Part model, mm, in its own coordinate system. A direction names the side the tool comes from. Coordinates: 2 decimals unless noted, no trailing zeros. Write each loop counter-clockwise with the first axis right and the second up, starting at its lowest first coordinate (ties: lowest second). Pieces come first, ordered by that corner, then holes. Notation, with made-up numbers: (25, 73.25) -> (64, 73.25) arc R27 cw to (64, 98.25) -> close; hole circle Ø9 at (27.5, -22.75). An arc over 180 degrees is marked (long way). Write item = value, one per line.
from build123d import *

# Parameters (mm, degrees)
SKETCH1_W           = 91
SKETCH1_H           = 24
BOSS_EXTRUDE1_DEPTH = 4
SKETCH2_R           = 1.675
CUT_EXTRUDE1_DEPTH  = 48.22552276
SKETCH3_W           = 91
SKETCH3_H           = 6
CUT_EXTRUDE2_DEPTH  = 2.5
SKETCH4_W           = 91
SKETCH4_H           = 4
BOSS_EXTRUDE2_DEPTH = 2.2
SKETCH5_W           = 91
SKETCH5_H           = 2
BOSS_EXTRUDE3_DEPTH = 17.62
SKETCH6_R           = 1.75
CUT_EXTRUDE3_DEPTH  = 55.464248824
SKETCH7_W           = 91
SKETCH7_H           = 24.2
SKETCH7_R           = 1.675
BOSS_EXTRUDE5_DEPTH = 2
SKETCH8_W           = 91
SKETCH8_H           = 6
BOSS_EXTRUDE6_DEPTH = 1
CHAMFER1_SIZE       = 0.7
FILLET1_R           = 3


with BuildPart() as part:
    # Sketch1 → Boss-Extrude1 (new body)
    with BuildSketch(Plane(origin=(0, 0, 0), x_dir=(1, 0, 0), z_dir=(0, 1, 0))):
        Rectangle(SKETCH1_W, SKETCH1_H)
    extrude(amount=BOSS_EXTRUDE1_DEPTH)

    # Sketch2 → Cut-Extrude1 (cut, through all)
    with BuildSketch(Plane(origin=(0, 4, 0), x_dir=(1, 0, 0), z_dir=(0, 1, 0))):
        with Locations(Location((-40.6, 3.5, 0), (0, 0, 270))):
            Circle(SKETCH2_R)
        with Locations(Location((-40.6, -9.95, 0), (0, 0, 270))):
            Circle(SKETCH2_R)
        with Locations(Location((40.6, 3.5, 0), (0, 0, 270))):
            Circle(SKETCH2_R)
        with Locations(Location((40.6, -9.95, 0), (0, 0, 270))):
            Circle(SKETCH2_R)
    extrude(amount=-CUT_EXTRUDE1_DEPTH, mode=Mode.SUBTRACT)

    # Sketch3 → Cut-Extrude2 (cut)
    with BuildSketch(Plane(origin=(0, 4, 0), x_dir=(1, 0, 0), z_dir=(0, 1, 0))):
        with Locations((0, -3.65)):
            Rectangle(SKETCH3_W, SKETCH3_H)
    extrude(amount=-CUT_EXTRUDE2_DEPTH, mode=Mode.SUBTRACT)

    # Sketch4 → Boss-Extrude2 (add)
    with BuildSketch(Plane(origin=(0, 0, -12), x_dir=(-1, 0, 0), z_dir=(0, 0, -1))):
        with Locations((0, 2)):
            Rectangle(SKETCH4_W, SKETCH4_H)
    extrude(amount=BOSS_EXTRUDE2_DEPTH)

    # Sketch5 → Boss-Extrude3 (add)
    with BuildSketch(Plane.XZ):
        with Locations((0, -13.2)):
            Rectangle(SKETCH5_W, SKETCH5_H)
    extrude(amount=BOSS_EXTRUDE3_DEPTH)

    # Sketch6 → Cut-Extrude3 (cut, through all)
    with BuildSketch(Plane.XY.offset(-12.2)):
        with Locations((-21.25, -10.12)):
            Circle(SKETCH6_R)
        with Locations((0, -10.12)):
            Circle(SKETCH6_R)
        with Locations((21.25, -10.12)):
            Circle(SKETCH6_R)
    extrude(amount=-CUT_EXTRUDE3_DEPTH, mode=Mode.SUBTRACT)

    # Sketch7 → Boss-Extrude5 (add)
    with BuildSketch(Plane.XZ):
        with Locations((0, -0.1)):
            Rectangle(SKETCH7_W, SKETCH7_H)
        with Locations(Location((40.6, 9.95, 0), (0, 0, 90))):
            Circle(SKETCH7_R, mode=Mode.SUBTRACT)
        with Locations(Location((40.6, -3.5, 0), (0, 0, 90))):
            Circle(SKETCH7_R, mode=Mode.SUBTRACT)
        with Locations(Location((-40.6, -3.5, 0), (0, 0, 90))):
            Circle(SKETCH7_R, mode=Mode.SUBTRACT)
        with Locations(Location((-40.6, 9.95, 0), (0, 0, 90))):
            Circle(SKETCH7_R, mode=Mode.SUBTRACT)
    extrude(amount=BOSS_EXTRUDE5_DEPTH)

    # Sketch8 → Boss-Extrude6 (add)
    with BuildSketch(Plane.XY.offset(12)):
        with Locations((0, 1)):
            Rectangle(SKETCH8_W, SKETCH8_H)
    extrude(amount=BOSS_EXTRUDE6_DEPTH)

    # Chamfer1
    chamfer1_edges = [part.edges().sort_by_distance(p)[0] for p in [
        (40.6, 4, 8.275),
        (-40.6, 4, -5.175),
        (40.6, 4, -5.175),
        (-40.6, 4, 8.275),
    ]]
    chamfer(chamfer1_edges, length=CHAMFER1_SIZE)

    # Fillet1
    fillet1_edges = [part.edges().sort_by_distance(p)[0] for p in [
        (0, -2, -12.2),
    ]]
    fillet(fillet1_edges, radius=FILLET1_R)


solid = part.part
Q1. Saw through at C-C on y = -10.12. Give the cut face in (x, z).
Model answer:
outline = (-45.5, -14.2) -> (-23, -14.2) -> (-23, -12.2) -> (-45.5, -12.2) -> close; (-19.5, -14.2) -> (-1.75, -14.2) -> (-1.75, -12.2) -> (-19.5, -12.2) -> close; (1.75, -14.2) -> (19.5, -14.2) -> (19.5, -12.2) -> (1.75, -12.2) -> close; (23, -14.2) -> (45.5, -14.2) -> (45.5, -12.2) -> (23, -12.2) -> close
Q2. Saw through at B-B on x = -40.6. Give the cut face in (y, z) (3 decimals), and give its area (3 significant figures).
Model answer:
outline = (-17.62, -14.2) -> (4, -14.2) -> (4, -5.875) -> (3.3, -5.175) -> (-2, -5.175) -> (-2, -9.2) arc R3 cw to (-5, -12.2) -> (-17.62, -12.2) -> close; (-2, -1.825) -> (3.3, -1.825) -> (4, -1.125) -> (4, 0.65) -> (1.5, 0.65) -> (1.5, 6.65) -> (4, 6.65) -> (4, 7.575) -> (3.3, 8.275) -> (-2, 8.275) -> close; (-2, 11.625) -> (3.3, 11.625) -> (4, 12.325) -> (4, 13) -> (-2, 13) -> close
area = 140 mm²
Q3. Pin check, flat tips, straight feed: pin 1 (2 mm diameter, centred on x = -34, z = -3, fed in from -Y); pin 2 (12 mm diameter, centred on x = 2.5, z = -10.5, fed in from -Y); pin 3 (3 mm diameter, centred on x = -22, z = 3.5, fed in from +Y); pin 4 (5.5 mm diameter, centred on x = 21.25, y = -10.12, fed in from +Z). Stop position of each tip, or through.
Model answer:
pin_1 = -2
pin_2 = -17.62
pin_3 = 1.5
pin_4 = -12.2
Q4. Saw through at A-A on z = 9.95. Give the cut face in (x, y) (3 decimals).
Model answer:
outline = (-45.5, -2) -> (-42.275, -2) -> (-42.275, 3.3) -> (-42.975, 4) -> (-45.5, 4) -> close; (-38.925, -2) -> (38.925, -2) -> (38.925, 3.3) -> (38.225, 4) -> (-38.225, 4) -> (-38.925, 3.3) -> close; (42.275, -2) -> (45.5, -2) -> (45.5, 4) -> (42.975, 4) -> (42.275, 3.3) -> close
Q5. Which spindle directions (+Z, -Z, +X, -X, +Y, -Y) get a long thin tool onto all of the face, cutting with end or side? Do faces 5 (the face through (-1, -7, -14.2)), 6 (the face through (-1, -2, 2)), 7 (the face through (-1, 3, 0.65)). Say none if no direction does.
Model answer:
face_5 = -Z, +X, -X, +Y, -Y
face_6 = +Z, +X, -X, -Y
face_7 = +X, -X, +Y
Q6. Probe line 1 (X direction, y = 1.7, z = -3.5) (3 decimals); line 2 (Z direction, x = -40.6, y = 1) (3 decimals); line 3 (Y direction, x = 21.25, z = -12.9). List the from-to ranges inside material, lowest first. Write a range as from..to.
Model answer:
line_1 = -45.5..-42.275, -38.925..38.925, 42.275..45.5
line_2 = -14.2..-5.175, -1.825..8.275, 11.625..13
line_3 = -17.62..-11.87, -8.37..4
Q7. Mould opens along Z. For faces 1 (the face through (-1, 4, 10)), 2 (the face through (0.64, -2.86, -11.3)), 3 (the face through (-1, 3, 6.65)), 4 (the face through (-39, 1, -4)) say: released by +Z, released by -Z, zero draft, split by the parting line, or undercut.
Model answer:
face_1 = zero draft
face_2 = released by +Z
face_3 = undercut
face_4 = undercut
Q8. Saw through at D-D on x = 0. Give the cut face in (y, z), and give its area (3 significant figures).
Model answer:
outline = (-17.62, -14.2) -> (-11.87, -14.2) -> (-11.87, -12.2) -> (-17.62, -12.2) -> close; (-8.37, -14.2) -> (4, -14.2) -> (4, 0.65) -> (1.5, 0.65) -> (1.5, 6.65) -> (4, 6.65) -> (4, 13) -> (-2, 13) -> (-2, -9.2) arc R3 cw to (-5, -12.2) -> (-8.37, -12.2) -> close
area = 174 mm²
